```python
from build123d import *

# Parameters (mm, degrees)
SKETCH001_W = 42
SKETCH001_H = 42
PAD_DEPTH   = 4.65


with BuildPart() as part:
    # Sketch001 → Pad (new body)
    with BuildSketch(Plane.XY):
        Rectangle(SKETCH001_W, SKETCH001_H)
        with BuildLine():
            Line((-16, -18.15), (16, -18.15))
            ThreePointArc((16, -18.15), (17.52028, -17.52028), (18.15, -16))
            Line((18.15, -16), (18.15, 16))
            ThreePointArc((18.15, 16), (17.52028, 17.52028), (16, 18.15))
            Line((16, 18.15), (-16, 18.15))
            ThreePointArc((-16, 18.15), (-17.52028, 17.52028), (-18.15, 16))
            Line((-18.15, 16), (-18.15, -16))
            ThreePointArc((-18.15, -16), (-17.52028, -17.52028), (-16, -18.15))
        make_face(mode=Mode.SUBTRACT)
    extrude(amount=-PAD_DEPTH)

    # SubtractivePipe: sweep along a path in Sketch002
    with BuildLine(Plane.XY) as subtractivepipe_path:
        Line((-16, -21), (16, -21))
        ThreePointArc((16, -21), (19.535534, -19.535534), (21, -16))
        Line((21, -16), (21, 16))
        ThreePointArc((21, 16), (19.535534, 19.535534), (16, 21))
        Line((16, 21), (-16, 21))
        ThreePointArc((-16, 21), (-19.535534, 19.535534), (-21, 16))
        Line((-21, 16), (-21, -16))
        ThreePointArc((-21, -16), (-19.535534, -19.535534), (-16, -21))
    # Sketch → SubtractivePipe (sweep, cut)
    with BuildSketch(Plane.XZ):
        Polygon((-21, 0), (-18.85, -2.15), (-18.85, -3.95), (-18.15, -4.65), (-18.15, 0), align=None)
    sweep(path=subtractivepipe_path.line, mode=Mode.SUBTRACT)


solid = part.part
```
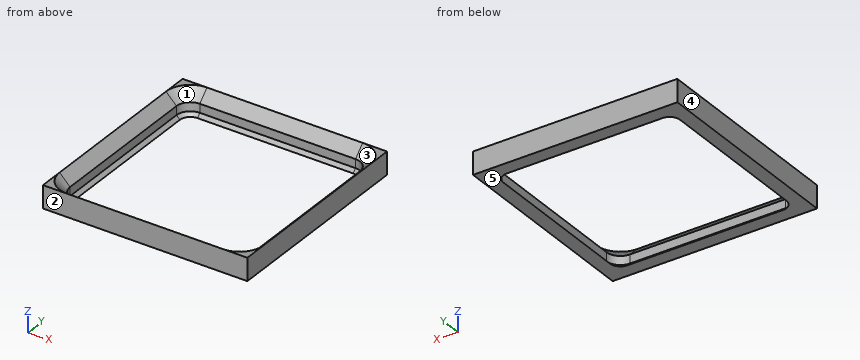
Read the model definition and answer for the solid it produces. Units are mm, in the model's axes. Face numbers are marked on the shaded views. A direction names the side the tool comes from. Coordinates: 2 decimals unless noted, no trailing zeros. Write each loop counter-clockwise with the first axis right and the second up, starting at its lowest first coordinate (ties: lowest second). Pieces come first, ordered by that corner, then holes. Notation, with made-up numbers: (-16.75, 14.25) -> (41.25, 14.25) arc R23 cw to (41.25, 43.25) -> close; hole circle Ø5 at (3.25, 15.25). An arc over 180 degrees is marked (long way). Answer as a JSON object with one key per item and string values.
Q1. A tool of negligible diameter and unlimited length cuts with its end or side. For the marked faces 1 and 2, from which of +Z, -Z, +X, -X, +Y, -Y can it reach the whole face along a straight path? Write none if from no direction.
The answers:
{"face 1": "+Z", "face 2": "+Z, -Z, +X, -X, -Y"}
Q2. The part is cut by section D-D on z = -3.15. Give the vertices of the cut face in (x, y).
The answers:
{"outline": "(-21, -21) -> (21, -21) -> (21, 21) -> (-21, 21) -> close; hole (-18.85, -16) arc R2.85 ccw to (-16, -18.85) -> (16, -18.85) arc R2.85 ccw to (18.85, -16) -> (18.85, 16) arc R2.85 ccw to (16, 18.85) -> (-16, 18.85) arc R2.85 ccw to (-18.85, 16) -> close"}
Q3. The part is cut by section A-A on y = 13. Give the vertices of the cut face in (x, z).
The answers:
{"outline": "(-21, -4.65) -> (-18.15, -4.65) -> (-18.85, -3.95) -> (-18.85, -2.15) -> (-21, 0) -> close; (18.15, -4.65) -> (21, -4.65) -> (21, 0) -> (18.85, -2.15) -> (18.85, -3.95) -> close"}
Q4. Consider line 1 (X direction, y = -5, z = -2.7); line 2 (Y direction, x = -5, z = -1.4). Determine where each line is inside the solid, lowest interval first. Write a range as [from, to].
The answers:
{"line 1": "x = [-21, -18.85], [18.85, 21]", "line 2": "y = [-21, -19.6], [19.6, 21]"}
Q5. The part is cut by section C-C on z = -1. Give the vertices of the cut face in (x, y).
The answers:
{"outline": "(-21, -21) -> (21, -21) -> (21, 21) -> (-21, 21) -> close; hole (-20, -16) arc R4 ccw to (-16, -20) -> (16, -20) arc R4 ccw to (20, -16) -> (20, 16) arc R4 ccw to (16, 20) -> (-16, 20) arc R4 ccw to (-20, 16) -> close"}
Q6. Determine the mould class of the marked faces 3, 4 and 5 for opening direction X: pulls with the +X half, pulls with the -X half, needs draft (parallel to the pull), parting line crosses it, or undercut.
The answers:
{"face 3": "undercut", "face 4": "pulls with the -X half", "face 5": "needs draft"}
